For this review, use the dimensioned drawing (mm, ordinates from the lowest corner) and the shaded views. Give positions to 0.01 mm unless a question says otherwise; leave off trailing zeros. Order: outer loops, then holes, each group sorted by start corner. A loop starts at its lowest first (then second) coordinate and runs counter-clockwise, first axis right, second up.
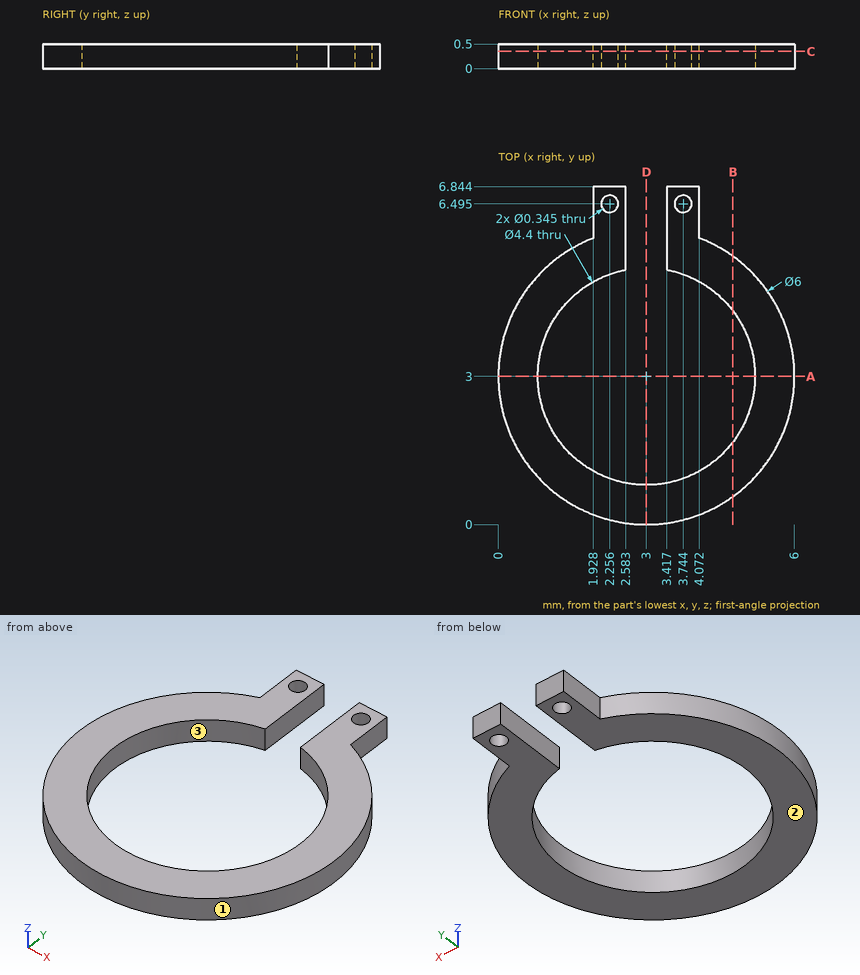
1. Draft analysis for pull direction Y (two halves, no side actions). For the marked faces 1, 2 and 3, state which applies: pulls with the +Y half, pulls with the -Y half, needs draft (parallel to the pull), parting line crosses it, or undercut.
Recorded:
face 1: parting line crosses it
face 2: needs draft
face 3: undercut
2. Take a section at B-B (x = 4.75). State the section outline as (y, z) points.
Recorded:
outline: (0.56, 0) - (1.67, 0) - (1.67, 0.5) - (0.56, 0.5) - close; (4.33, 0) - (5.44, 0) - (5.44, 0.5) - (4.33, 0.5) - close
3. Take a section at D-D (x = 3). State the section outline as (y, z) points.
Recorded:
outline: (0, 0) - (0.8, 0) - (0.8, 0.5) - (0, 0.5) - close
4. Take a section at A-A (y = 3). State the section outline as (x, z) points.
Recorded:
outline: (0, 0) - (0.8, 0) - (0.8, 0.5) - (0, 0.5) - close; (5.2, 0) - (6, 0) - (6, 0.5) - (5.2, 0.5) - close
5. Take a section at C-C (z = 0.35). State the section outline as (x, y) points (1 decimal).
Recorded:
outline: (1.9, 5.8) arc R3 ccw (long way) to (4.1, 5.8) - (4.1, 6.8) - (3.4, 6.8) - (3.4, 5.2) arc R2.2 cw (long way) to (2.6, 5.2) - (2.6, 6.8) - (1.9, 6.8) - close; hole circle Ø0.3 at (2.3, 6.5); hole circle Ø0.3 at (3.7, 6.5)
6. For line 1 along X through (y, z) = (6.5, 0.05); line 2 along X through (y, z) = (3, 0.45); line 3 along Y through (x, z) = (5, 0.25) (1 decimal), list the stretches that pass through material, from the lowest coordinate up.
Recorded:
line 1: x = 1.93 to 2.08, 2.43 to 2.58, 3.42 to 3.57, 3.92 to 4.07
line 2: x = 0 to 0.8, 5.2 to 6
line 3: y = 0.8 to 2.1, 3.9 to 5.2
